CAD build for the part. Positions are in the model's coordinates, mm. A direction names the side the tool comes from. Round coordinates to 2 decimals unless told otherwise and drop trailing zeros. Write each loop counter-clockwise with the first axis right and the second up, starting at its lowest first coordinate (ties: lowest second). Pieces come first, ordered by that corner, then holes. Notation, with made-up numbers: (-36, 20.25) - (-24, 20.25) arc R23 ccw to (-24, 53.25) - close; hole circle Ø7 at (-24.75, -12). An arc over 180 degrees is marked (long way). Put each result on its own line as item: value. Start each with the question number.
Item 1: Cut at C-C (z = 364.25). Give the cut face in (x, y), and give its area (3 significant figures).
Item 2: Drill centre lines: line 1 (Y direction, x = -90, z = 371.95); line 2 (Y direction, x = -81.25, z = 354.25); line 3 (X direction, y = -20, z = 371.6). Where is each one in solid material? Low to high. Write a range as from..to.
Item 3: Cut at D-D (x = -77.5). Give the cut face in (y, z).
Item 4: Cut at B-B (y = 20). Give the cut face in (x, z).
Item 5: Cut at A-A (x = -90). Give the cut face in (y, z).
Item 6: 3-axis set-ups, long thin cutter, end or side, ignore diameter. For faces 1 (the flat face through (-83, 0, 373.2)), 2 (the flat face through (-71.7, -32, 361)), 3 (the flat face through (-82, -30.3, 361)): which of +Z, -Z, +X, -X, +Y, -Y reach the whole face in a straight line?
Item 7: Pin check, flat tips, straight feed: pin 1 Ø1.5 at (x, y) = (-90.5, 19.5) entering from -Z; pin 2 Ø1.9 at (y, z) = (-32, 365) entering from +X; pin 3 Ø1.2 at (x, y) = (-90, -20) entering from +Z; pin 4 Ø3 at (y, z) = (24.5, 369) entering from +X. Stop position of each tip, or through.
Item 8: Mould opens along Y. For faces 4 (the flat face through (-83, -32.7, 362)), 5 (the flat face through (-94.7, 0, 362)), 6 (the flat face through (-92.3, 0, 361)) say: released by +Y, released by -Y, zero draft, split by the parting line, or undercut.
```python
from build123d import *

# Parameters (mm, degrees)
U_SKIRT_DEPTH                 = 18.2
SKETCH2_W                     = 24.7
SKETCH2_H                     = 65.4
TOP_PLATE_DEPTH               = 3
FILAMENT_PIN_HOLES_DEPTH      = 102.826420933
FILAMENT_PIN_HOLES_DEPTH_BACK = 102.826420933
SKETCH3_R                     = 1


with BuildPart() as part:
    # Sketch1 → U_skirt (new body)
    with BuildSketch(Plane.XY.offset(352)):
        Polygon((-94.7, -32.7), (-71.7, -32.7), (-71.7, -30.3), (-92.3, -30.3), (-92.3, 30.3), (-71.7, 30.3), (-71.7, 32.7), (-94.7, 32.7), align=None)
    extrude(amount=U_SKIRT_DEPTH)

    # Sketch2 → Top_plate (add)
    with BuildSketch(Plane.XY.offset(370.2)):
        with Locations((-82.35, 0)):
            Rectangle(SKETCH2_W, SKETCH2_H)
    extrude(amount=TOP_PLATE_DEPTH)

    # Sketch3 → Filament_pin_holes (cut, two sides: drawn at the far end of the back side and taken through both)
    with BuildSketch(Plane.XY.offset(370.2).offset(-FILAMENT_PIN_HOLES_DEPTH_BACK)):
        with Locations((-90, 20)):
            Circle(SKETCH3_R)
        with Locations((-90, -20)):
            Circle(SKETCH3_R)
    extrude(amount=FILAMENT_PIN_HOLES_DEPTH + FILAMENT_PIN_HOLES_DEPTH_BACK, mode=Mode.SUBTRACT)


solid = part.part
```
Output values:
1. outline: (-94.7, -32.7) - (-71.7, -32.7) - (-71.7, -30.3) - (-92.3, -30.3) - (-92.3, 30.3) - (-71.7, 30.3) - (-71.7, 32.7) - (-94.7, 32.7) - close
1. area: 256 mm2
2. line 1: -32.7..-21, -19..19, 21..32.7
2. line 2: -32.7..-30.3, 30.3..32.7
2. line 3: -94.7..-91, -89..-70
3. outline: (-32.7, 352) - (-30.3, 352) - (-30.3, 370.2) - (30.3, 370.2) - (30.3, 352) - (32.7, 352) - (32.7, 373.2) - (-32.7, 373.2) - close
4. outline: (-94.7, 352) - (-92.3, 352) - (-92.3, 370.2) - (-91, 370.2) - (-91, 373.2) - (-94.7, 373.2) - close; (-89, 370.2) - (-70, 370.2) - (-70, 373.2) - (-89, 373.2) - close
5. outline: (-32.7, 352) - (-30.3, 352) - (-30.3, 370.2) - (-21, 370.2) - (-21, 373.2) - (-32.7, 373.2) - close; (-19, 370.2) - (19, 370.2) - (19, 373.2) - (-19, 373.2) - close; (21, 370.2) - (30.3, 370.2) - (30.3, 352) - (32.7, 352) - (32.7, 373.2) - (21, 373.2) - close
6. face 1: +Z, +X, -X, +Y, -Y
6. face 2: -Z, +X, +Y, -Y
6. face 3: -Z, +X
7. pin 1: z = 370.2
7. pin 2: x = -71.7
7. pin 3: through
7. pin 4: x = -70
8. face 4: released by -Y
8. face 5: zero draft
8. face 6: undercut
